The model under review builds one solid part; all positions refer to its coordinate system, in mm. Round coordinates to 2 decimals unless told otherwise and drop trailing zeros. Write each loop counter-clockwise with the first axis right and the second up, starting at its lowest first coordinate (ties: lowest second). Pieces come first, ordered by that corner, then holes.
Item 1: Clearance check with a flat-ended pin moving along its axis: pin 1 Ø12 at (x, z) = (-290.5, -34.5) entering from -Y. State where the tip first meets the part, or that it passes through.
Item 2: Add section C-C (y = 24.5). Give the boundary of the cut face in (x, z), plus the area to 3 significant figures.
Item 3: Add section A-A (z = 0). Give the boundary of the cut face in (x, y), plus the area to 3 significant figures.
Item 4: Add section B-B (x = 0). Give the boundary of the cut face in (y, z).
Item 5: To check wall thickness, follow L1, parallel to Z at x = 0, y = 9; L2, parallel to Z at x = -81.5, y = 36; L3, parallel to X at y = 35, z = 243.5. State the ranges of each line that lie inside material, in increasing order.
```python
from build123d import *

# Parameters (mm, degrees)
F0_W     = 800
F0_H     = 800
F1_DEPTH = 40
F2_R     = 300
F3_DEPTH = 40


with BuildPart() as f1:
    # F0 (on Front) → F1 (new body)
    with BuildSketch(Plane.XZ):
        Rectangle(F0_W, F0_H)
    extrude(amount=-F1_DEPTH)

    # F2 (on face) → F3 (cut)
    with BuildSketch(Plane.XZ):
        Circle(F2_R)
    extrude(amount=-F3_DEPTH, mode=Mode.SUBTRACT)


solid = f1.part
```
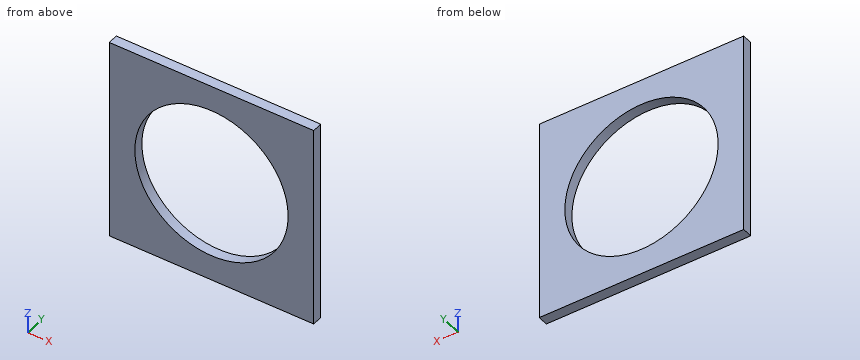
Numbers:
1. pin 1: passes through
2. outline: (-400, -400) - (400, -400) - (400, 400) - (-400, 400) - close; hole circle Ø600 at (0, 0)
2. area: 357,000 mm2
3. outline: (-400, 0) - (-300, 0) - (-300, 40) - (-400, 40) - close; (300, 0) - (400, 0) - (400, 40) - (300, 40) - close
3. area: 8,000 mm2
4. outline: (0, -400) - (40, -400) - (40, -300) - (0, -300) - close; (0, 300) - (40, 300) - (40, 400) - (0, 400) - close
5. L1: z = -400 to -300, 300 to 400
5. L2: z = -400 to -288.72, 288.72 to 400
5. L3: x = -400 to -175.24, 175.24 to 400
